from build123d import *

# Parameters (mm, degrees)
F1_ANGLE    = 180
F2_R        = 4
F2_R_2      = 2.25
F3_DEPTH    = 4.5
F4_DEPTH    = 8
F5_SIZE     = 1
F6_T1_DEPTH = 37.8922901759


# Not quite as in the source:
# - a fillet or chamfer that OpenCascade refuses, or shapes differently, is made with other operations: its cross-section is extruded or revolved along the edge and cut away or added


with BuildPart() as f1:
    # F0 (on Front) → F1 (revolve)
    with BuildSketch(Plane.XZ):
        Polygon((0, 12.5), (0, 10), (17, 10), (22, 12.8867513459), (22, 26), (14, 26), (14, 12.5), align=None)
    revolve(axis=Axis((14.5569612949, 0, 0), (1, 0, 0)), revolution_arc=F1_ANGLE)

    # F2 (on face) → F3 (cut)
    with BuildSketch(Plane(origin=(14, 0, 0), x_dir=(0, -1, 0), z_dir=(-1, 0, 0))):
        with Locations((20, 0)):
            Circle(F2_R)
        with Locations((20, 0)):
            Circle(F2_R_2, mode=Mode.SUBTRACT)
        with Locations((10, -17.3205080757)):
            Circle(F2_R)
        with Locations((10, -17.3205080757)):
            Circle(F2_R_2, mode=Mode.SUBTRACT)
        with Locations((10, 17.3205080757)):
            Circle(F2_R)
        with Locations((10, 17.3205080757)):
            Circle(F2_R_2, mode=Mode.SUBTRACT)
    extrude(amount=-F3_DEPTH, mode=Mode.SUBTRACT)

    # F4 (cut): faces of the model
    f4_faces = [f1.faces().sort_by_distance(p)[0] for p in [
        (14, -10, 17.3205080757),
        (14, -20, 0),
        (14, -10, -17.3205080757),
    ]]
    extrude(f4_faces, amount=-F4_DEPTH, mode=Mode.SUBTRACT)

    # F5
    f5_edges = [f1.edges().sort_by_distance(p)[0] for p in [
        (0, -12.5, 0),
        (14, -26, 0),
        (22, -26, 0),
    ]]
    chamfer(f5_edges, length=F5_SIZE)

    # F6: chamfer of 5 on 2 edges, made by hand

    # F6_s2 → F6_t1 (cut)
    with BuildSketch(Plane.YZ.offset(-0.946145088)):
        with BuildLine():
            Line((0, -20.3960780544), (-6.1904761905, -25.2522871149))
            ThreePointArc((-6.1904761905, -25.2522871149), (-3.188239959, -25.8037812338), (0, -26))
            Line((0, -26), (0, -20.3960780544))
        make_face()
        with BuildLine():
            Line((0, 20.3960780544), (-6.1904761905, 25.2522871149))
            ThreePointArc((-6.1904761905, 25.2522871149), (-3.188239959, 25.8037812338), (0, 26))
            Line((0, 26), (0, 20.3960780544))
        make_face()
    extrude(amount=F6_T1_DEPTH, mode=Mode.SUBTRACT)


solid = f1.part
Work out the finished part from the listing and answer in its coordinate system (mm). A direction names the side the tool comes from. Give positions to 0.01 mm unless a question says otherwise; leave off trailing zeros. Write each loop counter-clockwise with the first axis right and the second up, starting at its lowest first coordinate (ties: lowest second). Pieces come first, ordered by that corner, then holes. Notation, with made-up numbers: M 21,-33 L 54,-33 A23 ccw 54,0 Z; hole C -23,86.5 d11. An arc over 180 degrees is marked long. Answer as CSV lines item,"result".
Q1. Find the intervals of material crossed by probe 1 along X at (y, z) = (-15.25, -1); probe 2 along Z at (x, y) = (19.75, -3); probe 3 along Z at (x, y) = (4, -9), in increasing order. Write a range as [from, to].
A:
probe 1,"x = [14, 22]"
probe 2,"z = [-22.75, -11.19], [11.19, 22.75]"
probe 3,"z = [-8.67, -4.36], [4.36, 8.67]"
Q2. A cutting plane is placed at C-C on y = -10.5. Count the separate pieces of the cut face and the enclosed holes in it, plus the area to 3 significant figures.
A:
separate pieces,"3"
enclosed holes,"0"
area,"424 mm²"
Q3. A tool of negligible diameter and unlimited length cuts with its end or side. For faces 1 (the cylindrical face through (16.22, -7.05, 20.02)), 2 (the cylindrical face through (7.409, -12.497, 0.275)), 3 (the cylindrical face through (9, -10, 0)), from which of +Z, -Z, +X, -X, +Y, -Y can it reach the whole face along a straight path? Write none if from no direction.
A:
face 1,"-X"
face 2,"-X, -Y"
face 3,"+X, -X, +Y"
Q4. A cutting plane is placed at B-B on x = 16.25. Write down the section's boundary in (y, z), plus the area to 3 significant figures.
A:
outline,"M -6.19,-25.25 L 0,-20.4 L 0,-10 A10 cw 0,10 L 0,20.4 L -6.19,25.25 A26 ccw Z; hole C -20,0 d8; hole C -10,-17.32 d8; hole C -10,17.32 d8"
area,"718 mm²"
Q5. A cutting plane is placed at A-A on z = 0. Write down the section's boundary in (x, y), plus the area to 3 significant figures.
A:
outline,"M 0,-11.5 L 1,-12.5 L 14,-12.5 L 14,-16 L 18.5,-16 L 18.5,-17.75 L 22,-17.75 L 22,-12.89 L 17,-10 L 0,-10 Z; M 14,-25 L 15,-26 L 21,-26 L 22,-25 L 22,-22.25 L 18.5,-22.25 L 18.5,-24 L 14,-24 Z"
area,"103 mm²"
Q6. Given P1, Ø9, axis at y = -20.5, z = 2, coming from the -X side; P2, Ø7, axis at y = -10, z = -17.32, coming from the +X side; P3, Ø12, axis at x = 16, z = 2.5, coming from the -Y side; P4, Ø3, axis at x = 5.5, y = -12.5, coming from the +Z side, each flat-ended and moving along its own axis, determine where each tip first touches the part or whether it passes through.
A:
P1,"stops at x = 14"
P2,"stops at x = 22"
P3,"stops at y = -26"
P4,"stops at z = 5.94"
Q7. A cutting plane is placed at D-D on x = 10. Write down the section's boundary in (y, z).
A:
outline,"M 0,-12.5 L 0,-10 A10 cw 0,10 L 0,12.5 A12.5 ccw Z"
